Input: dimensioned drawing with shaded views. Units: mm. Origin: part minimum x, y, z. Give positions to 0.01 mm unless a question says otherwise; leave off trailing zeros. Loops run counter-clockwise (first coordinate to the right, second up) from the corner with the lowest first, then second, coordinate; pieces in that order, holes last. Notation, with made-up numbers: (-10.75, -26.5) -> (46.25, -26.5) arc R25 ccw to (46.25, -1.5) -> close; hole circle Ø5 at (9, 15.25). An arc over 180 degrees is marked (long way). Answer in a Markdown table with one row per item. Add a question column.
1) Line query: line 1 (Y direction, x = 8.5, z = 13.97); line 2 (Y direction, x = 20, z = 21); line 3 (Z direction, x = 17.5, y = 4.75). Output: solid intervals per line, ascending. Write a range as from..to.
2) Draft query along Z for the marked faces 1, 2 and 3. Return one class per face: +Z half, -Z half, draft (parallel to the pull), parting line (faces both ways), or undercut.
3) First-contact query: P1, Ø5, axis at x = 7.5, z = 24, coming from the +Y side; P2, Ø10, axis at y = 15, z = 23, coming from the -X side; P3, Ø6, axis at y = 3.5, z = 9.5, coming from the +X side (1 decimal); P4, Ø1.7, axis at x = 13.97, y = 8.466, coming from the -Z side. Flat tips, straight axial feed; report the tip coordinate or a pass-through.
4) Section query C-C (z = 24.97). Return the cut outline in (x, y).
5) Section query A-A (x = 13.97). Return the cut outline in (y, z), plus the area to 3 significant figures.
6) Section query B-B (z = 14). Return the cut outline in (x, y), plus the area to 3 significant figures.
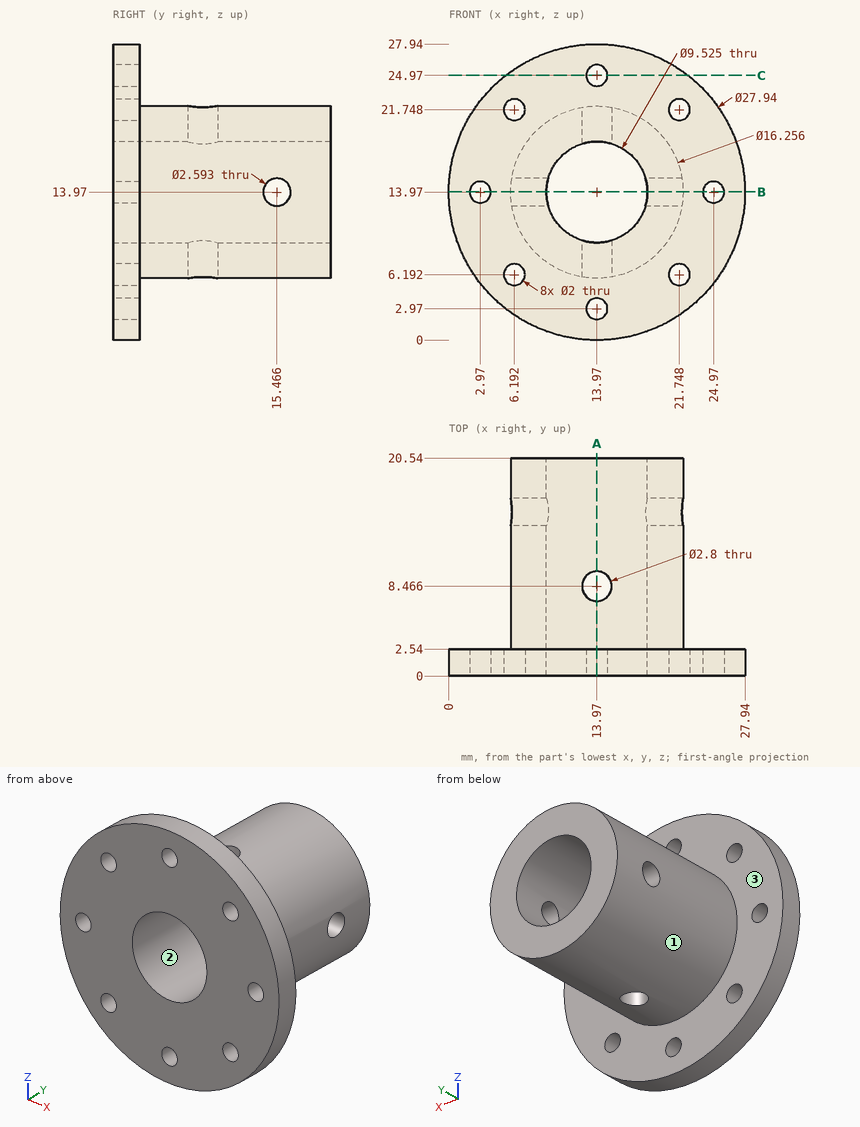
Evaluation:
| question | item | result |
|---|---|---|
| 1 | line 1 | 0..14.17, 16.76..20.54 |
| 1 | line 2 | 0..2.54 |
| 1 | line 3 | 6.65..10.77, 17.17..21.29 |
| 2 | face 1 | parting line |
| 2 | face 2 | undercut |
| 2 | face 3 | draft |
| 3 | P1 | y = 2.54 |
| 3 | P2 | x = 6.91 |
| 3 | P3 | x = 27.8 |
| 3 | P4 | through |
| 4 | outline | (5.36, 0) -> (12.97, 0) -> (12.97, 2.54) -> (5.36, 2.54) -> close; (14.97, 0) -> (22.58, 0) -> (22.58, 2.54) -> (14.97, 2.54) -> close |
| 5 | outline | (0, 0) -> (2.54, 0) -> (2.54, 1.97) -> (0, 1.97) -> close; (0, 3.97) -> (2.54, 3.97) -> (2.54, 5.84) -> (7.07, 5.84) -> (7.07, 9.21) -> (0, 9.21) -> close; (0, 18.73) -> (7.07, 18.73) -> (7.07, 22.1) -> (2.54, 22.1) -> (2.54, 23.97) -> (0, 23.97) -> close; (0, 25.97) -> (2.54, 25.97) -> (2.54, 27.94) -> (0, 27.94) -> close; (9.87, 5.84) -> (20.54, 5.84) -> (20.54, 9.21) -> (9.87, 9.21) -> close; (9.87, 18.73) -> (20.54, 18.73) -> (20.54, 22.1) -> (9.87, 22.1) -> close |
| 5 | area | 139 mm² |
| 6 | outline | (0, 0) -> (1.97, 0) -> (1.97, 2.54) -> (0, 2.54) -> close; (3.97, 0) -> (9.21, 0) -> (9.21, 14.17) -> (5.84, 14.17) -> (5.84, 2.54) -> (3.97, 2.54) -> close; (5.84, 16.76) -> (9.21, 16.76) -> (9.21, 20.54) -> (5.84, 20.54) -> close; (18.73, 0) -> (23.97, 0) -> (23.97, 2.54) -> (22.1, 2.54) -> (22.1, 14.17) -> (18.73, 14.17) -> close; (18.73, 16.76) -> (22.1, 16.76) -> (22.1, 20.54) -> (18.73, 20.54) -> close; (25.97, 0) -> (27.94, 0) -> (27.94, 2.54) -> (25.97, 2.54) -> close |
| 6 | area | 140 mm² |
